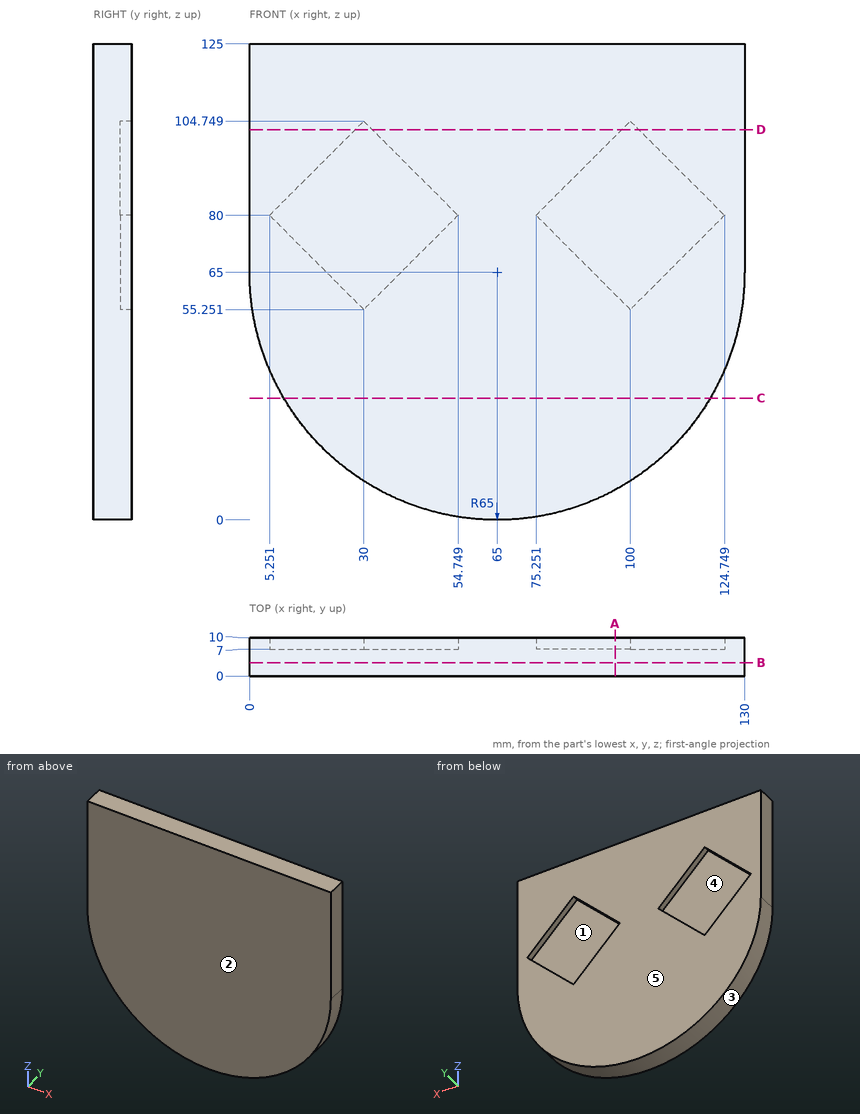
Answer from the drawing. Dimensions are ordinates in mm from the lowest x, y and z of the part. A direction names the side the tool comes from. Give positions to 0.01 mm unless a question says otherwise; leave off trailing zeros. Order: outer loops, then holes, each group sorted by start corner. A loop starts at its lowest first (then second) coordinate and runs counter-clockwise, first axis right, second up.
(1) Find section D-D (z = 102.5). Give the vertices of the cut face in (x, y).
(2) For a pull along X with two mould halves and no side action, classify the marked faces 3, 4 and 5 as released by +X, released by -X, zero draft, split by the parting line, or undercut.
(3) For the marked faces 1 and 2, determine the directions among +Z, -Z, +X, -X, +Y, -Y from which every point of the face is accessible in a straight line to the end or side of a thin tool.
(4) Straight lines are drawn through the part: L1, parallel to X at y = 8.5, z = 90.5; L2, parallel to X at y = 2.75, z = 64; L3, parallel to Y at x = 20, z = 66. For each, find the intervals that lie inside material, in ascending order.
(5) Find section B-B (y = 3.5). Give the vertices of the cut face in (x, z), plus the area to 3 significant figures.
(6) Given pin 1 (24.5 mm diameter, centred on x = 19.5, z = 81.5, fed in from +Y); pin 2 (3 mm diameter, centred on x = 28.5, z = 77.5, fed in from +Y); pin 3 (1 mm diameter, centred on x = 33, y = 8, fed in from -Z); pin 4 (3 mm diameter, centred on x = 35, y = 6, fed in from -Z), each flat-ended and moving along its own axis, determine where each tip first touches the part or whether it passes through.
(7) Find section C-C (z = 32). Give the vertices of the cut face in (x, y), plus the area to 3 significant figures.
(8) Find section A-A (x = 96). Give the vertices of the cut face in (y, z), plus the area to 3 significant figures.
Result sheet:
1. outline: (0, 0) - (130, 0) - (130, 10) - (102.25, 10) - (102.25, 7) - (97.75, 7) - (97.75, 10) - (32.25, 10) - (32.25, 7) - (27.75, 7) - (27.75, 10) - (0, 10) - close
2. face 3: split by the parting line
2. face 4: undercut
2. face 5: zero draft
3. face 1: +Y
3. face 2: +Z, -Z, +X, -X, -Y
4. L1: x = 0 to 15.75, 44.25 to 85.75, 114.25 to 130
4. L2: x = 0.01 to 129.99
4. L3: y = 0 to 7
5. outline: (0, 65) arc R65 ccw to (130, 65) - (130, 125) - (0, 125) - close
5. area: 14,400 mm2
6. pin 1: stops at y = 10
6. pin 2: stops at y = 7
6. pin 3: stops at z = 8.14
6. pin 4: stops at z = 6.58
7. outline: (9, 0) - (121, 0) - (121, 10) - (9, 10) - close
7. area: 1,120 mm2
8. outline: (0, 7.87) - (10, 7.87) - (10, 59.25) - (7, 59.25) - (7, 100.75) - (10, 100.75) - (10, 125) - (0, 125) - close
8. area: 1,050 mm2
